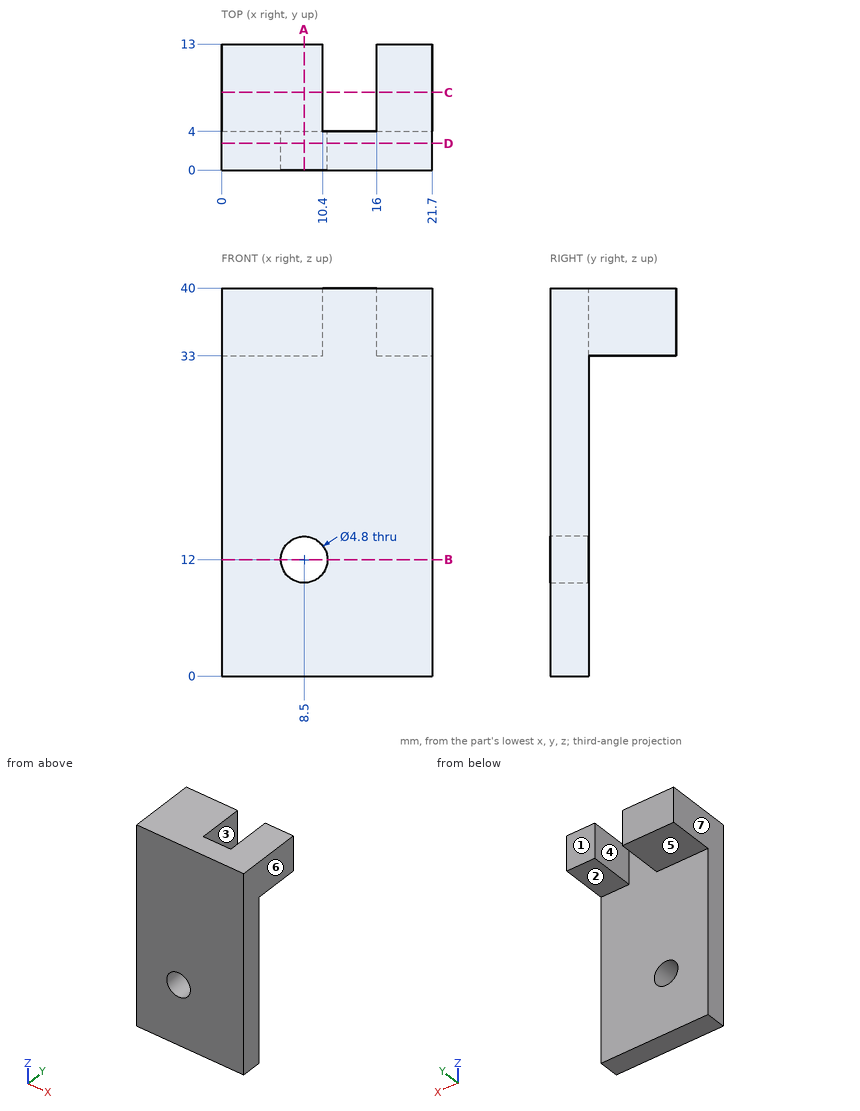
Check sheet for the drawn part. Datum: minimum x, y, z corner. Units: mm. A direction names the side the tool comes from. Round coordinates to 2 decimals unless told otherwise and drop trailing zeros. Order: outer loops, then holes, each group sorted by start corner. A loop starts at its lowest first (then second) coordinate and runs counter-clockwise, first axis right, second up. Notation, with made-up numbers: (48, 54.25) -> (97, 54.25) arc R26 cw to (97, 72.25) -> close; hole circle Ø4 at (-15, 26.5). An arc over 180 degrees is marked (long way). Put each result on its own line as item: value. Start each with the question number.
(1) Section check C-C (y = 8). Enter the section's corners in (x, z), then the cut area to 3 significant figures.
(2) Section check B-B (z = 12). Enter the section's corners in (x, y).
(3) Depth check by flat-ended pin: pin 1 Ø6 at (x, z) = (17.5, 23) entering from +Y; pin 2 Ø1.7 at (x, y) = (20, 7.5) entering from -Z. Enter the tip coordinate at first touch or a pass-through.
(4) Section check A-A (x = 8.5). Enter the section's corners in (y, z).
(5) Tool access check on the marked faces 1, 2 and 3. Record the directions out of +Z, -Z, +X, -X, +Y, -Y that give a thin tool (end or side, any length) a straight path to the whole face; none if there is none.
(6) Draft check along X on the marked faces 4, 5, 6 and 7. Enter one of: +X half, -X half, draft (parallel to the pull), parting line (faces both ways), or undercut.
(7) Material ranges on line 1 along X through (y, z) = (3, 12); line 2 along Z through (x, y) = (1.5, 11.5); line 3 along Y through (x, z) = (19, 20), recorded low to high.
(8) Section check D-D (y = 2.75). Enter the section's corners in (x, z).
Completed:
1. outline: (0, 33) -> (10.4, 33) -> (10.4, 40) -> (0, 40) -> close; (16, 33) -> (21.7, 33) -> (21.7, 40) -> (16, 40) -> close
1. area: 113 mm2
2. outline: (0, 0) -> (6.1, 0) -> (6.1, 4) -> (0, 4) -> close; (10.9, 0) -> (21.7, 0) -> (21.7, 4) -> (10.9, 4) -> close
3. pin 1: stops at y = 4
3. pin 2: stops at z = 33
4. outline: (0, 0) -> (4, 0) -> (4, 9.6) -> (0, 9.6) -> close; (0, 14.4) -> (4, 14.4) -> (4, 33) -> (13, 33) -> (13, 40) -> (0, 40) -> close
5. face 1: +Z, -Z, +X, -X, +Y
5. face 2: -Z, +X, -X, +Y
5. face 3: +Z, -Z, +Y
6. face 4: undercut
6. face 5: draft
6. face 6: +X half
6. face 7: -X half
7. line 1: x = 0 to 6.1, 10.9 to 21.7
7. line 2: z = 33 to 40
7. line 3: y = 0 to 4
8. outline: (0, 0) -> (21.7, 0) -> (21.7, 40) -> (0, 40) -> close; hole circle Ø4.8 at (8.5, 12)
